Model file for the job. Use its own axes, mm. A direction names the side the tool comes from. Give positions to 0.01 mm unless a question says otherwise; leave off trailing zeros. Write each loop counter-clockwise with the first axis right and the second up, starting at its lowest first coordinate (ties: lowest second). Pieces come first, ordered by that corner, then holes.
```python
from build123d import *

# Parameters (mm, degrees)
F0_W     = 40
F0_H     = 60
F1_DEPTH = 12
F2_W     = 30
F2_H     = 10
F3_DEPTH = 2
F4_R     = 5.5
F5_DEPTH = 20


with BuildPart() as f1:
    # F0 (on Top) → F1 (new body)
    with BuildSketch(Plane.XY):
        Rectangle(F0_W, F0_H)
    extrude(amount=F1_DEPTH)

    # F2 (on face) → F3 (cut)
    with BuildSketch(Plane.XZ.offset(30)):
        with Locations((0, 6)):
            Rectangle(F2_W, F2_H)
    extrude(amount=-F3_DEPTH, mode=Mode.SUBTRACT)

    # F4 (on face) → F5 (join)
    with BuildSketch(Plane(origin=(0, 30, 0), x_dir=(-1, 0, 0), z_dir=(0, 1, 0))):
        with Locations((0, 6)):
            Circle(F4_R)
    extrude(amount=F5_DEPTH)


solid = f1.part
```
1. Slice it at A-A, the plane x = 0. Write the cut outline in (y, z).
Calculated:
outline: (-30, 0) - (30, 0) - (30, 0.5) - (50, 0.5) - (50, 11.5) - (30, 11.5) - (30, 12) - (-30, 12) - (-30, 11) - (-28, 11) - (-28, 1) - (-30, 1) - close
2. Which spindle directions (+Z, -Z, +X, -X, +Y, -Y) get a long thin tool onto all of the face, cutting with end or side? Do faces 4 (the flat face through (0, 0, 0)), 5 (the flat face through (0, -28, 6)). Say none if no direction does.
Calculated:
face 4: -Z, +X, -X, +Y, -Y
face 5: -Y
3. Pin check, flat tip, straight feed: P1, Ø5, axis at x = -12, z = 9, coming from the +Y side. Stop position of the tip, or through.
Calculated:
P1: stops at y = 30
4. Slice it at B-B, the plane z = 6. Write the cut outline in (x, y), and give its area (3 significant figures).
Calculated:
outline: (-20, -30) - (-15, -30) - (-15, -28) - (15, -28) - (15, -30) - (20, -30) - (20, 30) - (5.5, 30) - (5.5, 50) - (-5.5, 50) - (-5.5, 30) - (-20, 30) - close
area: 2,560 mm2
5. Pull direction X, two halves, no side cores. Call faces 1 (the flat face through (-0.3, -30, 11.2)), 2 (the cylindrical face through (1.19, 39.86, 0.63)), 3 (the flat face through (15, -29, 6)): +X half, -X half, draft (parallel to the pull), parting line (faces both ways), or undercut.
Calculated:
face 1: draft
face 2: parting line
face 3: undercut
6. Probe probe 1 along Y at (x, z) = (-0.5, 8.5); probe 2 along Y at (x, z) = (14.5, 3); probe 3 along X at (y, z) = (36, 4.75). List the from-to ranges inside material, lowest first.
Calculated:
probe 1: y = -28 to 50
probe 2: y = -28 to 30
probe 3: x = -5.36 to 5.36
7. Slice it at C-C, the plane y = 35. Write the cut outline in (x, z).
Calculated:
outline: circle Ø11 at (0, 6)
